```python
from build123d import *

# Parameters (mm, degrees)
F0_W     = 53.881463
F0_H     = 51.368588
F1_DEPTH = 12.7
F2_R     = 5.08
F3_T     = -2.54


with BuildPart() as f1:
    # F0 (on Front) → F1 (new body, symmetric)
    with BuildSketch(Plane.XZ):
        with Locations((-2.059168, -1.109223)):
            Rectangle(F0_W, F0_H)
    extrude(amount=F1_DEPTH, both=True)

    # F2
    f2_edges = [f1.edges().sort_by_distance(p)[0] for p in [
        (24.881564, 0, -26.793517),
        (-28.999899, 0, -26.793517),
        (-28.999899, 12.7, -1.109223),
        (-2.059167, 12.7, -26.793517),
        (24.881564, 12.7, -1.109223),
    ]]
    fillet(f2_edges, radius=F2_R)

    # F3
    f3_openings = [f1.faces().sort_by_distance(p)[0] for p in [
        (-2.059167, -0.094363, 24.575071),
        (-2.059167, -12.7, -1.010586),
    ]]
    offset(amount=F3_T, openings=f3_openings)


solid = f1.part
```
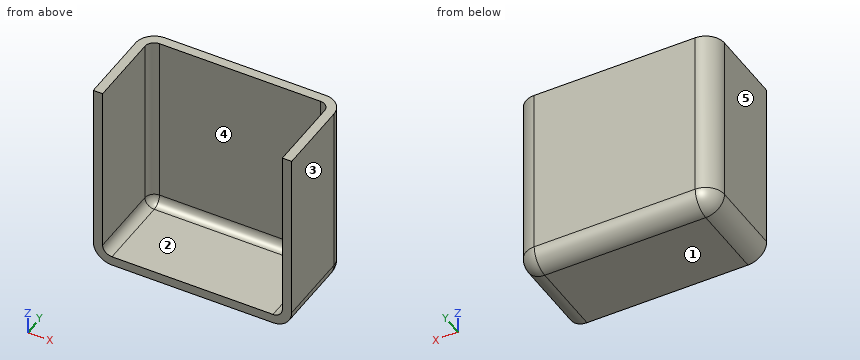
Can you work these out from the model? Positions are in its coordinate system, mm. Face numbers are marked on the shaded views. A direction names the side the tool comes from. Round coordinates to 2 decimals unless told otherwise and drop trailing zeros. Loops run counter-clockwise (first coordinate to the right, second up) from the corner with the lowest first, then second, coordinate; pieces in that order, holes last. Notation, with made-up numbers: (48.5, -19) -> (69.5, -19) arc R13 ccw to (69.5, 0) -> close; hole circle Ø5 at (53, 44). An arc over 180 degrees is marked (long way). Answer in a Markdown table with one row per item.
Item 1: On a 3-axis mill with a long thin cutter (end or side, diameter ignored), from which of +Z, -Z, +X, -X, +Y, -Y can I reach the whole of each face in a straight line? I mean the marked faces 1 and 2. Say none if no direction works.
Answer block:
| item | result |
|---|---|
| face 1 | -Z, +X, -X, +Y, -Y |
| face 2 | +Z, -Y |
Item 2: Will this pin go through, and if not, where does the flat tip stop? P1, Ø5, axis at x = 5, z = -9, coming from the -Y side.
Answer block:
| item | result |
|---|---|
| P1 | y = 10.16 |
Item 3: If I drill on probe 1 along X at (y, z) = (6.5, -16); probe 2 along Y at (x, z) = (-16, 19); probe 3 along X at (y, z) = (8, 3), over which ranges is the centre line in solid material (lowest first)?
Answer block:
| item | result |
|---|---|
| probe 1 | -29 to -26.46, 22.34 to 24.88 |
| probe 2 | 10.16 to 12.7 |
| probe 3 | -28.99 to -26.43, 22.31 to 24.87 |
Item 4: Suppose I cut it at B-B, the plane z = 5.5. List the corners of the cut face in (x, y) for me, plus the area to 3 significant figures.
Answer block:
| item | result |
|---|---|
| outline | (-29, -12.7) -> (-26.46, -12.7) -> (-26.46, 7.62) arc R2.54 cw to (-23.92, 10.16) -> (19.8, 10.16) arc R2.54 cw to (22.34, 7.62) -> (22.34, -12.7) -> (24.88, -12.7) -> (24.88, 7.62) arc R5.08 ccw to (19.8, 12.7) -> (-23.92, 12.7) arc R5.08 ccw to (-29, 7.62) -> close |
| area | 245 mm² |
Item 5: We'd pull the mould along X, two halves only. Please class the marked faces 3, 4 and 5: released by +X, released by -X, zero draft, split by the parting line, or undercut.
Answer block:
| item | result |
|---|---|
| face 3 | released by +X |
| face 4 | undercut |
| face 5 | released by -X |
Item 6: Suppose I cut it at C-C, the plane y = -3.5. List the corners of the cut face in (x, z) for me.
Answer block:
| item | result |
|---|---|
| outline | (-29, -21.71) arc R5.08 ccw to (-23.92, -26.79) -> (19.8, -26.79) arc R5.08 ccw to (24.88, -21.71) -> (24.88, 24.58) -> (22.34, 24.58) -> (22.34, -21.71) arc R2.54 cw to (19.8, -24.25) -> (-23.92, -24.25) arc R2.54 cw to (-26.46, -21.71) -> (-26.46, 24.58) -> (-29, 24.58) -> close |
Item 7: Suppose I cut it at A-A, the plane x = 19. List the corners of the cut face in (y, z) for me.
Answer block:
| item | result |
|---|---|
| outline | (-12.7, -26.79) -> (7.62, -26.79) arc R5.08 ccw to (12.7, -21.71) -> (12.7, 24.58) -> (10.16, 24.58) -> (10.16, -21.71) arc R2.54 cw to (7.62, -24.25) -> (-12.7, -24.25) -> close |
